Work out the finished part from the listing and answer in its coordinate system (mm). Face numbers are marked on the shaded views. Give positions to 0.01 mm unless a question says otherwise; leave off trailing zeros. Loops run counter-clockwise (first coordinate to the right, second up) from the corner with the lowest first, then second, coordinate; pieces in that order, holes last. Notation, with made-up numbers: (58.25, -24) -> (93.25, -24) arc R15 cw to (93.25, -19) -> close; hole circle Ø9 at (70.5, -2.75). An arc over 180 degrees is marked (long way). Answer as CSV lines item,"result". Start each with the question number.
1. Determine the mould class of the marked faces 1, 2, 3 and 4 for opening direction X: +X half, -X half, draft (parallel to the pull), parting line (faces both ways), or undercut.
2. Find section C-C, the plane y = -0.5. Give the vertices of the cut face in (x, z).
3. Find the intervals of material crossed by line 1 along X through (y, z) = (5.6, 0); line 2 along X through (y, z) = (5.8, 0); line 3 along Y through (x, z) = (-3.25, 0.25), in increasing order.
4. Find section D-D, the plane y = 5.25. Give the vertices of the cut face in (x, z), and give its area (3 significant figures).
5. Find section A-A, the plane y = -2.25. Give the vertices of the cut face in (x, z).
6. Find section B-B, the plane x = 0. Give the vertices of the cut face in (y, z).
7. Flat-ended cylindrical pins translate along their axes: pin 1 Ø4 at (x, y) = (-2.5, -1.5) entering from -Z; pin 2 Ø1.4 at (x, z) = (0, 0) entering from -Y; pin 3 Ø0.5 at (x, z) = (0, -4) entering from -Y. Find the tip coordinate at first contact, or state that the pin passes through.
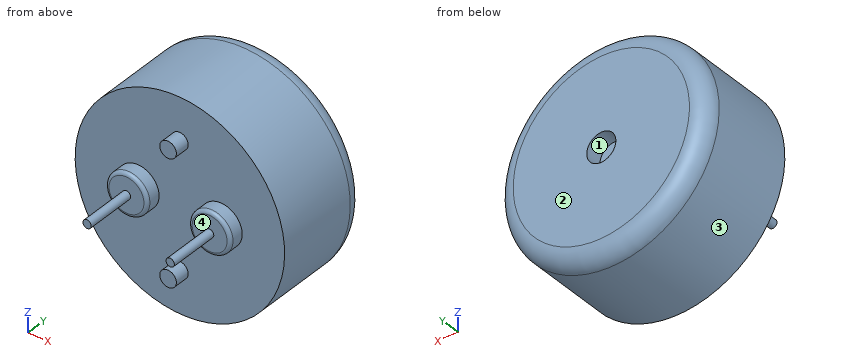
from build123d import *

# Parameters (mm, degrees)
SKETCH_1_R          = 6.3
SKETCH_1_R_2        = 1.25
SKETCH_1_R_3        = 0.5
SKETCH_1_R_4        = 0.25
SKETCH_1_R_5        = 0.875244423
EXTRUDE_1_DEPTH     = 6
FILLET_1_R          = 1
CUT_EXTRUDE_START   = 6
SKETCH_1_3_R        = 0.875244423
CUT_EXTRUDE_1_DEPTH = 1
SKETCH_1_4_R        = 1.25
SKETCH_1_4_R_2      = 0.25
SKETCH_1_4_R_3      = 0.5
EXTRUDE_2_DEPTH     = 0.9
FILLET_2_R          = 0.2
EXTRUDE_START       = -0.9
SKETCH_1_5_R        = 0.25
EXTRUDE_3_DEPTH     = 3


with BuildPart() as part:
    # Эскиз1 → Бобышка-Вытянуть1 (new body)
    # profile 1 of 8: a face of its own
    with BuildSketch(Plane(origin=(0, 0, 0), x_dir=(1, 0, 0), z_dir=(0, 1, 0))):
        with Locations(Location((0, 0, 0), (0, 0, 270))):
            Circle(SKETCH_1_R)
        with Locations((-2.5, 0)):
            Circle(SKETCH_1_R_2, mode=Mode.SUBTRACT)
        with Locations((2.5, 0)):
            Circle(SKETCH_1_R_2, mode=Mode.SUBTRACT)
        with Locations((0, 3.75)):
            Circle(SKETCH_1_R_3, mode=Mode.SUBTRACT)
        with Locations((0, -3.75)):
            Circle(SKETCH_1_R_3, mode=Mode.SUBTRACT)
    # profile 2 of 8: a face of its own
    with BuildSketch(Plane(origin=(0, 0, 0), x_dir=(1, 0, 0), z_dir=(0, 1, 0))):
        with Locations((-2.5, 0)):
            Circle(SKETCH_1_R_2)
        with Locations((-2.5, 0)):
            Circle(SKETCH_1_R_4, mode=Mode.SUBTRACT)
    # profile 3 of 8: a face of its own
    with BuildSketch(Plane(origin=(0, 0, 0), x_dir=(1, 0, 0), z_dir=(0, 1, 0))):
        with Locations((-2.5, 0)):
            Circle(SKETCH_1_R_4)
    # profile 4 of 8: a face of its own
    with BuildSketch(Plane(origin=(0, 0, 0), x_dir=(1, 0, 0), z_dir=(0, 1, 0))):
        with Locations((2.5, 0)):
            Circle(SKETCH_1_R_2)
        with Locations((2.5, 0)):
            Circle(SKETCH_1_R_4, mode=Mode.SUBTRACT)
    # profile 5 of 8: a face of its own
    with BuildSketch(Plane(origin=(0, 0, 0), x_dir=(1, 0, 0), z_dir=(0, 1, 0))):
        with Locations((2.5, 0)):
            Circle(SKETCH_1_R_4)
    # profile 6 of 8: a face of its own
    with BuildSketch(Plane(origin=(0, 0, 0), x_dir=(1, 0, 0), z_dir=(0, 1, 0))):
        with Locations((0, 3.75)):
            Circle(SKETCH_1_R_3)
    # profile 7 of 8: a face of its own
    with BuildSketch(Plane(origin=(0, 0, 0), x_dir=(1, 0, 0), z_dir=(0, 1, 0))):
        with Locations((0, -3.75)):
            Circle(SKETCH_1_R_3)
    # profile 8 of 8: a face of its own
    with BuildSketch(Plane(origin=(0, 0, 0), x_dir=(1, 0, 0), z_dir=(0, 1, 0))):
        Circle(SKETCH_1_R_5)
    extrude(amount=EXTRUDE_1_DEPTH)

    # Скругление1
    fillet_1_edges = [part.edges().sort_by_distance(p)[0] for p in [
        (0, 6, -6.3),
    ]]
    fillet(fillet_1_edges, radius=FILLET_1_R)

    # Эскиз1<3> → Вырез-Вытянуть1 (cut)
    with BuildSketch(Plane(origin=(0, 0, 0), x_dir=(1, 0, 0), z_dir=(0, 1, 0)).offset(CUT_EXTRUDE_START)):
        with Locations(Location((0, 0, 0), (0, 0, 270))):
            Circle(SKETCH_1_3_R)
    extrude(amount=-CUT_EXTRUDE_1_DEPTH, mode=Mode.SUBTRACT)

    # Эскиз1<4> → Бобышка-Вытянуть2 (add)
    # profile 1 of 6: a face of its own
    with BuildSketch(Plane(origin=(0, 0, 0), x_dir=(1, 0, 0), z_dir=(0, 1, 0))):
        with Locations(Location((-2.5, 0, 0), (0, 0, 270))):
            Circle(SKETCH_1_4_R)
        with Locations((-2.5, 0)):
            Circle(SKETCH_1_4_R_2, mode=Mode.SUBTRACT)
    # profile 2 of 6: a face of its own
    with BuildSketch(Plane(origin=(0, 0, 0), x_dir=(1, 0, 0), z_dir=(0, 1, 0))):
        with Locations(Location((0, -3.75, 0), (0, 0, 270))):
            Circle(SKETCH_1_4_R_3)
    # profile 3 of 6: a face of its own
    with BuildSketch(Plane(origin=(0, 0, 0), x_dir=(1, 0, 0), z_dir=(0, 1, 0))):
        with Locations(Location((2.5, 0, 0), (0, 0, 270))):
            Circle(SKETCH_1_4_R)
        with Locations((2.5, 0)):
            Circle(SKETCH_1_4_R_2, mode=Mode.SUBTRACT)
    # profile 4 of 6: a face of its own
    with BuildSketch(Plane(origin=(0, 0, 0), x_dir=(1, 0, 0), z_dir=(0, 1, 0))):
        with Locations((2.5, 0)):
            Circle(SKETCH_1_4_R_2)
    # profile 5 of 6: a face of its own
    with BuildSketch(Plane(origin=(0, 0, 0), x_dir=(1, 0, 0), z_dir=(0, 1, 0))):
        with Locations((-2.5, 0)):
            Circle(SKETCH_1_4_R_2)
    # profile 6 of 6: a face of its own
    with BuildSketch(Plane(origin=(0, 0, 0), x_dir=(1, 0, 0), z_dir=(0, 1, 0))):
        with Locations(Location((0, 3.75, 0), (0, 0, 270))):
            Circle(SKETCH_1_4_R_3)
    extrude(amount=-EXTRUDE_2_DEPTH)

    # Скругление2
    fillet_2_edges = [part.edges().sort_by_distance(p)[0] for p in [
        (2.5, -0.9, -1.25),
        (-2.5, -0.9, -1.25),
    ]]
    fillet(fillet_2_edges, radius=FILLET_2_R)

    # Эскиз1<5> → Бобышка-Вытянуть3 (add)
    with BuildSketch(Plane(origin=(0, 0, 0), x_dir=(1, 0, 0), z_dir=(0, 1, 0)).offset(EXTRUDE_START)):
        with Locations(Location((-2.5, 0, 0), (0, 0, 270))):
            Circle(SKETCH_1_5_R)
        with Locations(Location((2.5, 0, 0), (0, 0, 270))):
            Circle(SKETCH_1_5_R)
    extrude(amount=-EXTRUDE_3_DEPTH)


solid = part.part
Resolved:
1,face 1,"undercut"
1,face 2,"draft"
1,face 3,"parting line"
1,face 4,"undercut"
2,outline,"circle Ø2.5 at (-2.5, 0); circle Ø1 at (0, -3.75); circle Ø1 at (0, 3.75); circle Ø2.5 at (2.5, 0)"
3,line 1,"x = -6.1 to -0.88, 0.88 to 6.1"
3,line 2,"x = -5.9 to -0.88, 0.88 to 5.9"
3,line 3,"y = -0.9 to 6"
4,outline,"circle Ø12.54 at (0, 0); hole circle Ø1.75 at (0, 0)"
4,area,"121 mm^2"
5,outline,"circle Ø0.5 at (-2.5, 0); circle Ø0.5 at (2.5, 0)"
6,outline,"(-0.9, -4.25) -> (0, -4.25) -> (0, -6.3) -> (5, -6.3) arc R1 ccw to (6, -5.3) -> (6, -0.88) -> (5, -0.88) -> (5, 0.88) -> (6, 0.88) -> (6, 5.3) arc R1 ccw to (5, 6.3) -> (0, 6.3) -> (0, 4.25) -> (-0.9, 4.25) -> (-0.9, 3.25) -> (0, 3.25) -> (0, -3.25) -> (-0.9, -3.25) -> close"
7,pin 1,"stops at z = -6.19"
7,pin 2,"stops at y = 0"
7,pin 3,"stops at y = -0.9"
